Print and shaded views of the part. All mm, measured from the part's lowest x, y and z. A direction names the side the tool comes from. Round coordinates to 2 decimals unless told otherwise and drop trailing zeros. Loops run counter-clockwise (first coordinate to the right, second up) from the corner with the lowest first, then second, coordinate; pieces in that order, holes last. Notation, with made-up numbers: (34.5, 28.25) - (62.5, 28.25) arc R18 ccw to (62.5, 33.25) - close; hole circle Ø10 at (13, -15). An arc over 180 degrees is marked (long way). Use one line per item in the form item = value.
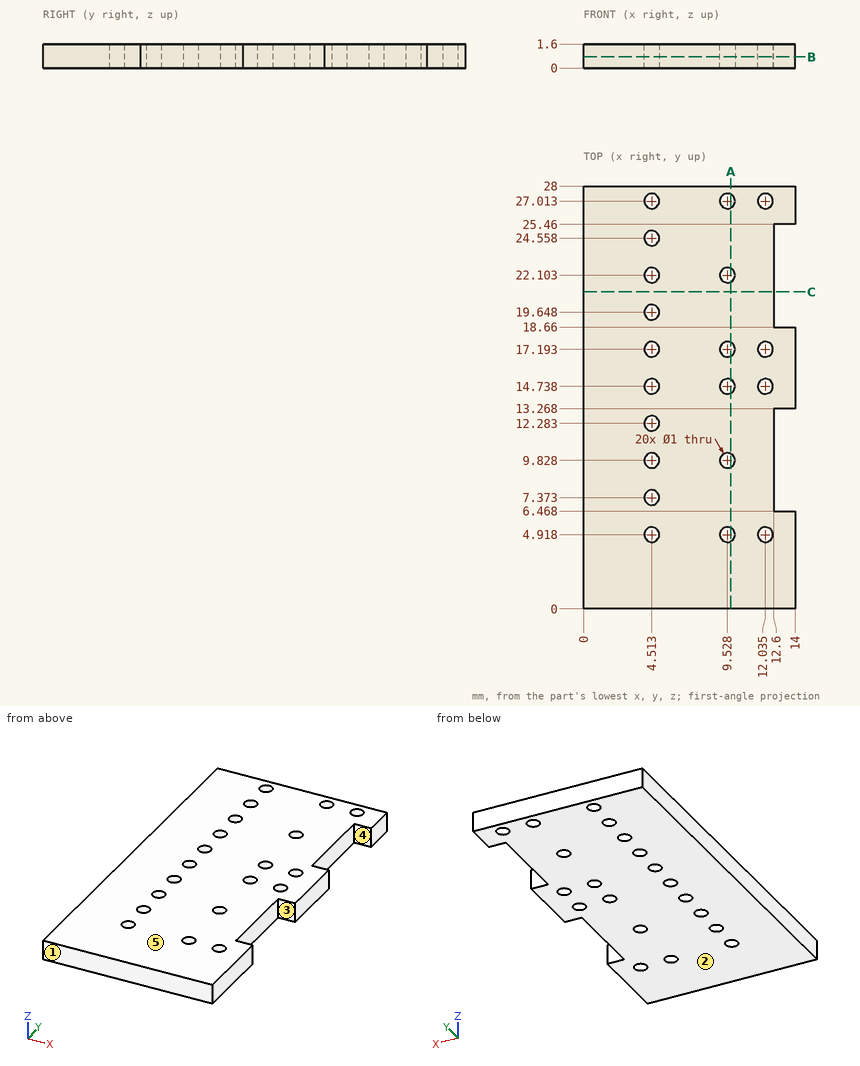
1) Tool access for the marked faces 4 and 5: list every direction of +Z, -Z, +X, -X, +Y, -Y with a clear straight run to the whole face (end or side of a thin tool).
Report:
face_4 = +Z, -Z, +X
face_5 = +Z, +X, -X, +Y, -Y
2) Slice it at C-C (y = 21). Write the cut outline in (x, z).
Report:
outline = (0, 0) - (12.6, 0) - (12.6, 1.6) - (0, 1.6) - close
3) Flat gauge pins, fed straight in: pin 1 (0.7 mm diameter, centred on x = 13, z = 0.5, fed in from -Y); pin 2 (0.5 mm diameter, centred on y = 9.5, z = 1, fed in from +X). Where does each tip first touch, or does it go through?
Report:
pin_1 = 0
pin_2 = 12.6
4) Drill centre lines: probe 1 along X at (y, z) = (5, 0.5) (1 decimal); probe 2 along X at (y, z) = (22.5, 0.3) (1 decimal); probe 3 along X at (y, z) = (24.5, 0.55). Where is each one in solid material? Low to high.
Report:
probe_1 = 0 to 4, 5 to 9, 10 to 11.5, 12.5 to 14
probe_2 = 0 to 4.2, 4.8 to 9.2, 9.8 to 12.6
probe_3 = 0 to 4.02, 5.01 to 12.6
5) Two-plate mould, pull along Y, no slides. Class the marked faces 1, 2 and 3: +Y half, -Y half, draft (parallel to the pull), parting line (faces both ways), or undercut.
Report:
face_1 = -Y half
face_2 = draft
face_3 = undercut
6) Slice it at A-A (x = 9.75). Write the cut outline in (y, z) (1 decimal).
Report:
outline = (0, 0) - (4.5, 0) - (4.5, 1.6) - (0, 1.6) - close; (5.4, 0) - (9.4, 0) - (9.4, 1.6) - (5.4, 1.6) - close; (10.3, 0) - (14.3, 0) - (14.3, 1.6) - (10.3, 1.6) - close; (15.2, 0) - (16.7, 0) - (16.7, 1.6) - (15.2, 1.6) - close; (17.6, 0) - (21.7, 0) - (21.7, 1.6) - (17.6, 1.6) - close; (22.6, 0) - (26.6, 0) - (26.6, 1.6) - (22.6, 1.6) - close; (27.5, 0) - (28, 0) - (28, 1.6) - (27.5, 1.6) - close
7) Slice it at B-B (z = 0.75). State how many separate pieces and enclosed holes the cut face has, plus the area to 3 significant figures.
Report:
separate_pieces = 1
enclosed_holes = 20
area = 357 mm^2
